Can you work these out from the model? Positions are in its coordinate system, mm. A direction names the side the tool comes from. Give positions to 0.01 mm unless a question says otherwise; leave off trailing zeros. Loops run counter-clockwise (first coordinate to the right, second up) from the corner with the lowest first, then second, coordinate; pieces in that order, holes last. Notation, with made-up numbers: (7.5, 62.5) -> (40.5, 62.5) arc R25 ccw to (40.5, 101.5) -> close; hole circle Ø6 at (86, -18.5). An arc over 180 degrees is marked (long way). Return JSON: item names as keys, results as strings. Group by question number.
Q1. Suppose I cut it at B-B, the plane z = 3.95. Please give me the cut outline in (x, y), and give its area (3 significant figures).
Q2. Will these pins go through, and if not, where does the flat tip stop? pin 1 (2 mm diameter, centred on x = -2, z = 2.5, fed in from -Y); pin 2 (0.7 mm diameter, centred on x = -0.5, y = 0.5, fed in from -Z).
Q3. Thinking about a two-plate mould opening in Y: for faces 4 (the flat face through (-1.65, 0, 1)), 5 (the flat face through (0, -1.3, 0)), 6 (the cylindrical face through (-3.546, 0.058, 2.169)), 7 (the cylindrical face through (2.952, 5.084, 2.169)), which applies, pulls with the +Y half, pulls with the -Y half, needs draft (parallel to the pull), parting line crosses it, or undercut?
Q4. Which directions (+Z, -Z, +X, -X, +Y, -Y) give clear straight access to the entire face, cutting with the end or side of a thin tool? Please do faces 1 (the flat face through (0, 1.1, 1)), 2 (the cylindrical face through (-0.027, -5.516, 2.169)), 3 (the cylindrical face through (0.027, 5.516, 2.169)).
Q5. Suppose I cut it at A-A, the plane z = 1.6. Please give me the cut outline in (x, y).
Q6. I need wall thicknesses on line 1 along Y through (x, z) = (0.5, 1.9); line 2 along Z through (x, y) = (0, 0.5); line 3 along Y through (x, z) = (-2.25, 0.3). Which ranges of each line are inside material? Lowest first, please. Write a range as [from, to].
```python
from build123d import *

# Parameters (mm, degrees)
SKETCH023_W  = 3.3
SKETCH023_H  = 2.2
PAD017_DEPTH = 2.5
PAD023_DEPTH = 5.5
FILLET_R     = 1.1


with BuildPart() as clone_button_hole_v:
    # Sketch023 → Pad017 (new body)
    with BuildSketch(Plane.XY):
        Rectangle(SKETCH023_W, SKETCH023_H)
    extrude(amount=PAD017_DEPTH)


with BuildPart() as cut_button_med_v_final:
    # Sketch044 → Pad023 (new body)
    with BuildSketch(Plane(origin=(0, 0, 0), x_dir=(0, 1, 0), z_dir=(0, 0, 1))):
        with BuildLine():
            ThreePointArc((4.124817, 3.4), (0, 3.546467), (-4.124817, 3.4))
            ThreePointArc((-4.124817, 3.4), (-5.094844, 2.941111), (-5.500001, 1.947441))
            ThreePointArc((-5.500001, 1.947441), (-5.515851, 0), (-5.5, -1.947441))
            ThreePointArc((-5.5, -1.947441), (-5.094843, -2.94111), (-4.124817, -3.4))
            ThreePointArc((-4.124817, -3.4), (0, -3.546467), (4.124817, -3.4))
            ThreePointArc((4.124817, -3.4), (5.094843, -2.94111), (5.5, -1.947441))
            ThreePointArc((5.5, -1.947441), (5.515851, 0), (5.500001, 1.947441))
            ThreePointArc((5.500001, 1.947441), (5.094844, 2.941111), (4.124817, 3.4))
        make_face()
    extrude(amount=PAD023_DEPTH)

    # Fillet
    fillet_edges = [cut_button_med_v_final.edges().sort_by_distance(p)[0] for p in [
        (-3.546467, 0, 5.5),
        (-2.941111, -5.094844, 5.5),
        (0, -5.515851, 5.5),
        (2.94111, -5.094843, 5.5),
        (3.546467, 0, 5.5),
        (2.94111, 5.094843, 5.5),
        (0, 5.515851, 5.5),
        (-2.941111, 5.094844, 5.5),
    ]]
    fillet(fillet_edges, radius=FILLET_R)

    # Cut008: cut Clone (button hole v)
    add(clone_button_hole_v.part, mode=Mode.SUBTRACT)


solid = cut_button_med_v_final.part
```
Ans:
{
 "1": {"outline": "(-3.4, -4.12) arc R1.48 ccw to (-1.95, -5.5) arc R119.64 ccw to (1.95, -5.5) arc R1.48 ccw to (3.4, -4.12) arc R58.15 ccw to (3.4, 4.12) arc R1.48 ccw to (1.95, 5.5) arc R119.64 ccw to (-1.95, 5.5) arc R1.48 ccw to (-3.4, 4.12) arc R58.15 ccw to start", "area": "74.6 mm^2"},
 "2": {"pin 1": "stops at y = -5.51", "pin 2": "stops at z = 2.5"},
 "3": {"face 4": "undercut", "face 5": "needs draft", "face 6": "parting line crosses it", "face 7": "pulls with the +Y half"},
 "4": {"face 1": "-Z", "face 2": "+Z, -Z, -Y", "face 3": "+Z, -Z, +Y"},
 "5": {"outline": "(-3.4, -4.12) arc R1.48 ccw to (-1.95, -5.5) arc R119.64 ccw to (1.95, -5.5) arc R1.48 ccw to (3.4, -4.12) arc R58.15 ccw to (3.4, 4.12) arc R1.48 ccw to (1.95, 5.5) arc R119.64 ccw to (-1.95, 5.5) arc R1.48 ccw to (-3.4, 4.12) arc R58.15 ccw to start; hole (-1.65, -1.1) -> (1.65, -1.1) -> (1.65, 1.1) -> (-1.65, 1.1) -> close"},
 "6": {"line 1": "y = [-5.51, -1.1], [1.1, 5.51]", "line 2": "z = [2.5, 5.5]", "line 3": "y = [-5.46, 5.46]"}
}
